Check sheet for the modelled part. Datum: model origin and axes. Units: mm. A direction names the side the tool comes from. Round coordinates to 2 decimals unless told otherwise and drop trailing zeros. Write each loop counter-clockwise with the first axis right and the second up, starting at its lowest first coordinate (ties: lowest second). Pieces come first, ordered by that corner, then holes.
Item 1: Depth check by flat-ended pin: pin 1 (0.6 mm diameter, centred on x = 0.5, z = -2, fed in from -Y). Enter the tip coordinate at first touch or a pass-through.
Item 2: Section check D-D, the plane x = -3.95. Record the cut outline in (y, z).
Item 3: Set-up check for faces 1 (the flat face through (-3.48, 2.63, 0.45)), 2 (the flat face through (0.246, 2.869, 0.276)), 3 (the flat face through (0.2, -0.5, -0.9)): record each of +Z, -Z, +X, -X, +Y, -Y from which the full face is reachable in a straight line by a thin tool's end or side.
Item 4: Release check for a two-part mould opening along Y. For faces 4 (the flat face through (-2, 1, 0)), 5 (the flat face through (0.25, -0.89, -0.01)), 6 (the flat face through (0.5, 1, 1)), 7 (the flat face through (-2, 6, 0)) record: pulls with the +Y half, pulls with the -Y half, needs draft (parallel to the pull), parting line crosses it, or undercut.
Item 5: Section check A-A, the plane x = -2.55. Record the cut outline in (y, z), plus the area to 3 significant figures.
Item 6: Section check C-C, the plane y = -1.5. Record the cut outline in (x, z).
Item 7: Material ranges on line 1 along X through (y, z) = (-1.5, 3.5); line 2 along X through (y, z) = (1, 0.5); line 3 along Y through (x, z) = (0.2, -1.25), recorded low to high.
Item 8: Section check B-B, the plane z = 2.25. Record the cut outline in (x, y).
Autodesk Inventor part; units mm, degrees
ref_plane "YZ Plane" through (0, 0, 0) normal (1, 0, 0) x (0, 1, 0)
ref_plane "XZ Plane" through (0, 0, 0) normal (0, 1, 0) x (-1, 0, 0)
ref_plane "XY Plane" through (0, 0, 0) normal (0, 0, 1) x (1, 0, 0)
sketch "Szkic1" plane through (0, 0, 0) normal (1, 0, 0) x (0, 1, 0)
  line L0 (6, 4) -> (-4, 4)
  line L1 (-4, 4) -> (-4, -3)
  line L2 (-4, -3) -> (6, -3)
  line L3 (6, -3) -> (6, 4)
  point P0 (0, 0)
  dimension "d0" = 10
  dimension "d1" = 7
extrude "Wyciągnięcie proste1" add sketch "Szkic1" against normal blind 5
sketch "Szkic2" plane through (0, 0, 0) normal (1, 0, 0) x (0, 0, -1)
  line L0 (-4, -4) -> (3, -4)
  line L1 (3, -4) -> (3, 6)
  line L2 (3, 6) -> (-4, 6)
  line L3 (-4, 6) -> (-4, -4)
  line L4 (-4, 6) -> (3, 6) construction
  line L5 (3, 6) -> (3, -4) construction
  line L6 (3, -4) -> (-4, -4) construction
  line L7 (-4, -4) -> (-4, 6) construction
  line L8 (2.4838, -2.5) -> (1.2755, -2.5)
  line L9 (1.2755, -2.5) -> (-1.2828, 0.7561)
  line L10 (-1.2828, 0.7561) -> (-1.6912, 0.2966)
  line L11 (-1.6912, 0.2966) -> (-1.6912, -2.5)
  line L12 (-1.6912, -2.5) -> (-2.6216, -2.5)
  line L13 (-2.6216, -2.5) -> (-2.6216, 4.5)
  line L14 (-2.6216, 4.5) -> (-1.6912, 4.5)
  line L15 (-1.6912, 4.5) -> (-1.6912, 1.2836)
  line L16 (-1.6912, 1.2836) -> (1.1791, 4.5)
  line L17 (1.1791, 4.5) -> (2.3136, 4.5)
  line L18 (2.3136, 4.5) -> (-0.5851, 1.3744)
  line L19 (-0.5851, 1.3744) -> (2.4838, -2.5)
  point P0 (0, 0)
  point P1 (-0.5, 6)
  point P2 (-0.5, 6)
  point P3 (3, 1)
  point P4 (3, 1)
  dimension "d4" = 10
  dimension "d5" = 7
extrude "Wyciągnięcie proste2" add sketch "Szkic2" along normal blind 0.5 contours L8 L9 L10 L11 L12 L13 L14 L15 L16 L17 L18 L19
sketch "Szkic3" plane through (0, -4, -3) normal (0, 0, -1) x (-1, 0, 0)
  line L0 (2, 7) -> (2, 3)
  line L1 (2, 3) -> (5, 3.75)
  line L2 (2, 7) -> (5, 6.25)
  line L3 (5, 6.25) -> (5, 3.75)
  line L4 (5, 10) -> (5, 0)
  point P0 (0, 4)
  point P1 (5, 5)
  point P2 (5, 5)
  point P3 (2, 5)
  point P4 (5, 5)
  dimension "d8" = 4
  dimension "d12" = 3
  dimension "d13" = 2.5
extrude "Wyciągnięcie proste3" cut sketch "Szkic3" against normal blind 10
properties part number "literka"
Values found:
1. pin 1: stops at y = -2.5
2. outline: (-4, -3) - (-0.51, -3) - (-0.51, 4) - (-4, 4) - close; (2.51, -3) - (6, -3) - (6, 4) - (2.51, 4) - close
3. face 1: +Z, -Z
3. face 2: +X, +Y
3. face 3: -Z, +X
4. face 4: undercut
4. face 5: pulls with the -Y half
4. face 6: needs draft
4. face 7: pulls with the +Y half
5. outline: (-4, -3) - (-0.86, -3) - (-0.86, 4) - (-4, 4) - close; (2.86, -3) - (6, -3) - (6, 4) - (2.86, 4) - close
5. area: 43.9 mm2
6. outline: (-5, -3) - (0, -3) - (0, -1.69) - (0.5, -1.69) - (0.5, -0.49) - (0, -0.49) - (0, 1.69) - (0.5, 1.69) - (0.5, 2.62) - (0, 2.62) - (0, 4) - (-5, 4) - close
7. line 1: x = -5 to 0
7. line 2: x = -2 to 0.5
7. line 3: y = -2.47 to -0.94, 3.35 to 4.5
8. outline: (-5, -4) - (0, -4) - (0, -2.5) - (0.5, -2.5) - (0.5, 4.5) - (0, 4.5) - (0, 6) - (-5, 6) - (-5, 2.25) - (-2, 3) - (-2, -1) - (-5, -0.25) - close
